For this review, take the finished solid that the model builds, in its own axes (mm). Round coordinates to 2 decimals unless told otherwise and drop trailing zeros. Order: outer loops, then holes, each group sorted by start corner. A loop starts at its lowest first (then second) coordinate and runs counter-clockwise, first axis right, second up. Notation, with made-up numbers: M 8,31.5 L 44,31.5 A30 cw 44,67.5 Z; hole C 15,17 d3. An arc over 180 degrees is marked long. Write item = value, one per line. Start each with the question number.
from build123d import *

# Parameters (mm, degrees)
ESQUISSE1_W                = 400
ESQUISSE1_H                = 107
BOSS_EXTRU_1_DEPTH         = 5
ESQUISSE2_W                = 5
ESQUISSE2_H                = 16
ENL_V_MAT_EXTRU_1_DEPTH    = 5
R_P_TITION_LIN_AIRE1_COUNT = 4
R_P_TITION_LIN_AIRE1_PITCH = 32
SYM_TRIE1_COPY_1_SKETCH_W  = 5
SYM_TRIE1_COPY_1_SKETCH_H  = 16
SYM_TRIE1_COPY_1_DEPTH     = 5
SYM_TRIE1_COPY_2_SKETCH_W  = 5
SYM_TRIE1_COPY_2_SKETCH_H  = 16
SYM_TRIE1_COPY_2_DEPTH     = 5
SYM_TRIE1_COPY_3_SKETCH_W  = 5
SYM_TRIE1_COPY_3_SKETCH_H  = 16
SYM_TRIE1_COPY_3_DEPTH     = 5
ESQUISSE3_W                = 16
ESQUISSE3_H                = 5
ENL_V_MAT_EXTRU_2_DEPTH    = 5
R_P_TITION_LIN_AIRE2_COUNT = 13
R_P_TITION_LIN_AIRE2_PITCH = 32
ESQUISSE4_W                = 40
ESQUISSE4_H                = 70
ENL_V_MAT_EXTRU_3_DEPTH    = 10
R_P_TITION_LIN_AIRE3_COUNT = 5
R_P_TITION_LIN_AIRE3_PITCH = 75


with BuildPart() as part:
    # Esquisse1 → Boss.-Extru.1 (new body)
    with BuildSketch(Plane.XY):
        with Locations((200, -53.5)):
            Rectangle(ESQUISSE1_W, ESQUISSE1_H)
    extrude(amount=BOSS_EXTRU_1_DEPTH)

    # Esquisse2 → Enlèv. mat.-Extru.1 (cut)
    with BuildSketch(Plane.XY.offset(5)):
        with Locations((2.5, -99)):
            Rectangle(ESQUISSE2_W, ESQUISSE2_H)
    enl_v_mat_extru_1 = extrude(amount=-ENL_V_MAT_EXTRU_1_DEPTH, mode=Mode.SUBTRACT)

    # Répétition linéaire1: Enlèv. mat.-Extru.1 ×4
    with Locations(*[(0, i * R_P_TITION_LIN_AIRE1_PITCH, 0) for i in range(1, R_P_TITION_LIN_AIRE1_COUNT)]):
        add(enl_v_mat_extru_1, mode=Mode.SUBTRACT)

    # Symétrie1: Enlèv. mat.-Extru.1 across plane
    add(enl_v_mat_extru_1.mirror(Plane.ZY.offset(-200)), mode=Mode.SUBTRACT)

    # Symétrie1 copy 1 sketch → Symétrie1 copy 1 (cut)
    with BuildSketch(Plane(origin=(400, 32, 5), x_dir=(-1, 0, 0), z_dir=(0, 0, 1))):
        with Locations((2.5, 99)):
            Rectangle(SYM_TRIE1_COPY_1_SKETCH_W, SYM_TRIE1_COPY_1_SKETCH_H)
    extrude(amount=-SYM_TRIE1_COPY_1_DEPTH, mode=Mode.SUBTRACT)

    # Symétrie1 copy 2 sketch → Symétrie1 copy 2 (cut)
    with BuildSketch(Plane(origin=(400, 64, 5), x_dir=(-1, 0, 0), z_dir=(0, 0, 1))):
        with Locations((2.5, 99)):
            Rectangle(SYM_TRIE1_COPY_2_SKETCH_W, SYM_TRIE1_COPY_2_SKETCH_H)
    extrude(amount=-SYM_TRIE1_COPY_2_DEPTH, mode=Mode.SUBTRACT)

    # Symétrie1 copy 3 sketch → Symétrie1 copy 3 (cut)
    with BuildSketch(Plane(origin=(400, 96, 5), x_dir=(-1, 0, 0), z_dir=(0, 0, 1))):
        with Locations((2.5, 99)):
            Rectangle(SYM_TRIE1_COPY_3_SKETCH_W, SYM_TRIE1_COPY_3_SKETCH_H)
    extrude(amount=-SYM_TRIE1_COPY_3_DEPTH, mode=Mode.SUBTRACT)

    # Esquisse3 → Enlèv. mat.-Extru.2 (cut)
    with BuildSketch(Plane.XY.offset(5)):
        with Locations((8, -104.5)):
            Rectangle(ESQUISSE3_W, ESQUISSE3_H)
    enl_v_mat_extru_2 = extrude(amount=-ENL_V_MAT_EXTRU_2_DEPTH, mode=Mode.SUBTRACT)

    # Répétition linéaire2: Enlèv. mat.-Extru.2 ×13
    with Locations(*[(i * R_P_TITION_LIN_AIRE2_PITCH, 0, 0) for i in range(1, R_P_TITION_LIN_AIRE2_COUNT)]):
        add(enl_v_mat_extru_2, mode=Mode.SUBTRACT)

    # Esquisse4 → Enlèv. mat.-Extru.3 (cut)
    with BuildSketch(Plane.XY.offset(5)):
        with Locations((50, -52)):
            Rectangle(ESQUISSE4_W, ESQUISSE4_H)
    enl_v_mat_extru_3 = extrude(amount=-ENL_V_MAT_EXTRU_3_DEPTH, mode=Mode.SUBTRACT)

    # Répétition linéaire3: Enlèv. mat.-Extru.3 ×5
    with Locations(*[(i * R_P_TITION_LIN_AIRE3_PITCH, 0, 0) for i in range(1, R_P_TITION_LIN_AIRE3_COUNT)]):
        add(enl_v_mat_extru_3, mode=Mode.SUBTRACT)


solid = part.part
(1) For line 1 along X through (y, z) = (-26.5, 1.3); line 2 along X through (y, z) = (-37, 2.7); line 3 along Y through (x, z) = (194, 2.15), list the stretches that pass through material, from the lowest coordinate up.
(2) Insertion check: pin 1 (2 mm diameter, centred on y = -95.5, z = 2.5, fed in from -X); pin 2 (2.5 mm diameter, centred on x = 203, z = 3, fed in from -Y); pin 3 (1.5 mm diameter, centred on y = -104, z = 1.5, fed in from +X). Each pin has a flat end and moves straight along its axis. Give the tip position at first contact, or say it passes through.
(3) We need section B-B, the plane y = -70.5. Write out the cut boundary in (x, z).
(4) We need section A-A, the plane x = 137. Write out the cut boundary in (y, z), then the cut area to 3 significant figures.
(5) We need section D-D, the plane z = 4. State how many separate pieces and enclosed holes the cut face has, then the cut area to 3 significant figures.
(6) We need section C-C, the plane x = 56.5. Write out the cut boundary in (y, z).
Values:
q1.line_1 = 0 to 30, 70 to 105, 145 to 180, 220 to 255, 295 to 330, 370 to 400
q1.line_2 = 5 to 30, 70 to 105, 145 to 180, 220 to 255, 295 to 330, 370 to 395
q1.line_3 = -102 to -87, -17 to 0
q2.pin_1 = 5
q2.pin_2 = -102
q2.pin_3 = 384
q3.outline = M 5,0 L 30,0 L 30,5 L 5,5 Z; M 70,0 L 105,0 L 105,5 L 70,5 Z; M 145,0 L 180,0 L 180,5 L 145,5 Z; M 220,0 L 255,0 L 255,5 L 220,5 Z; M 295,0 L 330,0 L 330,5 L 295,5 Z; M 370,0 L 395,0 L 395,5 L 370,5 Z
q4.outline = M -102,0 L -87,0 L -87,5 L -102,5 Z; M -17,0 L 0,0 L 0,5 L -17,5 Z
q4.area = 160 mm²
q5.separate_pieces = 1
q5.enclosed_holes = 5
q5.area = 27,200 mm²
q6.outline = M -107,0 L -87,0 L -87,5 L -107,5 Z; M -17,0 L 0,0 L 0,5 L -17,5 Z
